```python
from build123d import *

# Parameters (mm, degrees)
EXTRUDE_1_DEPTH                    = 20
SKETCH_5_R                         = 0.7
EXTRUDE_3_DEPTH                    = 4
CUT_EXTRUDE_1_DEPTH                = 8.5
SKETCH_7_R                         = 0.65
EXTRUDE_4_DEPTH                    = 6.7
CHAMFER_1_SIZE                     = 0.3
PATTERN_LINEAR_2_COUNT             = 4
PATTERN_LINEAR_2_PITCH             = 5
PATTERN_LINEAR_3_COUNT             = 4
PATTERN_LINEAR_3_PITCH             = 5
CHAMFER_1_OF_PATTERN_LINEAR_3_SIZE = 0.3
EXTRUDE_5_DEPTH                    = 0.5
EXTRUDE_6_DEPTH                    = 0.5
CUT_EXTRUDE_2_REACH                = 28.613
SKETCH_10_W                        = 0.5
SKETCH_10_H                        = 8.5


with BuildPart() as part:
    # Эскиз1 → Вытянуть1 (new body)
    with BuildSketch(Plane(origin=(0, 0, 0), x_dir=(0, -1, 0), z_dir=(1, 0, 0))):
        Polygon((-9, 0), (-9, -0.5), (-12, 0), (-12, 8), (0, 8), (0, 0), align=None)
    extrude(amount=EXTRUDE_1_DEPTH)

    # Эскиз5 → Вытянуть3 (add)
    with BuildSketch(Plane(origin=(0, 8, -8), x_dir=(1, 0, 0), z_dir=(0, 0, 1))):
        with Locations((2.5, -6.5)):
            Circle(SKETCH_5_R)
    extrude_3 = extrude(amount=-EXTRUDE_3_DEPTH)

    # Эскиз6 → Вырез-Вытянуть1 (cut)
    with BuildSketch(Plane(origin=(0, 12, 0), x_dir=(1, 0, 0), z_dir=(0, 1, 0))):
        with BuildLine():
            Line((0, 6.5), (0, 1))
            Line((0, 1), (5, 1))
            Line((5, 1), (5, 6.5))
            ThreePointArc((5, 6.5), (2.5, 7.3), (0, 6.5))
        make_face()
    cut_extrude_1 = extrude(amount=-CUT_EXTRUDE_1_DEPTH, mode=Mode.SUBTRACT)

    # Эскиз7 → Вытянуть4 (add)
    with BuildSketch(Plane(origin=(0, 3.5, 0), x_dir=(1, 0, 0), z_dir=(0, 1, 0))):
        with Locations(Location((2.5, 4, 0), (0, 0, 90))):
            Circle(SKETCH_7_R)
    extrude_4 = extrude(amount=EXTRUDE_4_DEPTH)

    # Фаска1
    chamfer_1_edges = [part.edges().sort_by_distance(p)[0] for p in [
        (2.5, 10.2, -3.35),
    ]]
    chamfer(chamfer_1_edges, length=CHAMFER_1_SIZE)

    # Линейный массив2: Вытянуть3, Вырез-Вытянуть1 ×4
    with Locations(*[(i * PATTERN_LINEAR_2_PITCH, 0, 0) for i in range(1, PATTERN_LINEAR_2_COUNT)]):
        add(extrude_3)
        add(cut_extrude_1, mode=Mode.SUBTRACT)

    # Линейный массив3: Вытянуть4 ×4
    with Locations(*[(i * PATTERN_LINEAR_3_PITCH, 0, 0) for i in range(1, PATTERN_LINEAR_3_COUNT)]):
        add(extrude_4)

    # Фаска1 of Линейный массив3
    chamfer_1_of_pattern_linear_3_edges = [part.edges().sort_by_distance(p)[0] for p in [
        (7.5, 10.2, -3.35),
        (12.5, 10.2, -3.35),
        (17.5, 10.2, -3.35),
    ]]
    chamfer(chamfer_1_of_pattern_linear_3_edges, length=CHAMFER_1_OF_PATTERN_LINEAR_3_SIZE)

    # Эскиз8 → Вытянуть5 (add)
    with BuildSketch(Plane(origin=(20, 0, 0), x_dir=(0, 0, -1), z_dir=(1, 0, 0))):
        Polygon((0, 12), (8, 12), (8, 0), (0, 0), (0, 9), (-0.5, 9), align=None)
    extrude(amount=EXTRUDE_5_DEPTH)

    # Эскиз9 → Вытянуть6 (add)
    with BuildSketch(Plane.ZY):
        Polygon((-8, 12), (0, 12), (0.5, 9), (0, 9), (0, 0), (-8, 0), align=None)
    extrude(amount=EXTRUDE_6_DEPTH)

    # Эскиз10 → Вырез-Вытянуть2 (cut, up to next)
    with BuildSketch(Plane(origin=(0, 12, 0), x_dir=(1, 0, 0), z_dir=(0, 1, 0)), mode=Mode.PRIVATE) as cut_extrude_2_sk1:
        with Locations((20.25, 3.75)):
            Rectangle(SKETCH_10_W, SKETCH_10_H)
    cut_extrude_2_tool1 = extrude(cut_extrude_2_sk1.sketch, amount=-CUT_EXTRUDE_2_REACH, mode=Mode.PRIVATE) & part.part
    # Эскиз10 → Вырез-Вытянуть2 (cut, up to next)
    with BuildSketch(Plane(origin=(0, 12, 0), x_dir=(1, 0, 0), z_dir=(0, 1, 0)), mode=Mode.PRIVATE) as cut_extrude_2_sk2:
        with Locations((-0.25, 3.75)):
            Rectangle(SKETCH_10_W, SKETCH_10_H)
    cut_extrude_2_tool2 = extrude(cut_extrude_2_sk2.sketch, amount=-CUT_EXTRUDE_2_REACH, mode=Mode.PRIVATE) & part.part
    add(cut_extrude_2_tool1.solids().sort_by_distance((20.25, 12, -3.75))[0], mode=Mode.SUBTRACT)
    add(cut_extrude_2_tool2.solids().sort_by_distance((-0.25, 12, -3.75))[0], mode=Mode.SUBTRACT)


solid = part.part
```
Part model, mm, in its own coordinate system. A direction names the side the tool comes from. Give positions to 0.01 mm unless a question says otherwise; leave off trailing zeros. Order: outer loops, then holes, each group sorted by start corner. A loop starts at its lowest first (then second) coordinate and runs counter-clockwise, first axis right, second up. Notation, with made-up numbers: M 47,80.25 L 102,80.25 A25 cw 102,114.25 Z; hole C 56.25,48 d6. An arc over 180 degrees is marked long. Use a Markdown table: item, result. Add a question column.
(1) Drop flat-ended pins along their axis: P1, Ø1, axis at x = 15.5, y = 5.5, coming from the +Z side; P2, Ø0.8, axis at x = 12.5, z = -4, coming from the +Y side; P3, Ø1, axis at x = 13, z = -9.5, coming from the -Y side; P4, Ø5, axis at x = 5, z = -5, coming from the +Y side. Give the stop position or say it passes through.
(2) 3-axis set-ups, long thin cutter, end or side, ignore diameter. For faces 1 (the face through (10, 8, -1)), 2 (the face through (12.5, 7.8, -7.3)), 3 (the face through (13.147, 1.232, -9.972)): which of +Z, -Z, +X, -X, +Y, -Y reach the whole face in a straight line?
(3) Saw through at A-A, the plane y = 3.75. Give the cut face in (x, z), and give its area (3 significant figures).
(4) Saw through at D-D, the plane y = 1.5. Give the cut face in (x, z), and give its area (3 significant figures).
(5) Mould opens along X. For faces 4 (the face through (2.823, 0.879, -9.972)), 5 (the face through (10.1, 12, -0.5)), 6 (the face through (20, 3, -5)), 7 (the face through (7.3, 6.66, -4.62)) say: +X half, -X half, draft (parallel to the pull), parting line (faces both ways), or undercut.
(6) Probe line 1 along Z through (x, y) = (12.5, 7.25); line 2 along X through (y, z) = (4, -3.75); line 3 along Z through (x, y) = (19, 2.5). List the from-to ranges inside material, lowest first. Write a range as [from, to].
(7) Saw through at C-C, the plane z = -11. Give the cut face in (x, y), and give its area (3 significant figures).
(8) Saw through at B-B, the plane x = 2.5. Give the cut face in (y, z).
Answer key:
| question | item | result |
|---|---|---|
| 1 | P1 | z = 0 |
| 1 | P2 | y = 10.2 |
| 1 | P3 | y = 0.8 |
| 1 | P4 | y = 12 |
| 2 | face 1 | +X, -X, +Y |
| 2 | face 2 | +Y |
| 2 | face 3 | -Z |
| 3 | outline | M 0,-8 L 20,-8 L 20,-6.5 A4.31 cw 15,-6.5 A4.31 cw 10,-6.5 A4.31 cw 5,-6.5 A4.31 cw 0,-6.5 Z; M 0,-1 L 20,-1 L 20,0 L 0,0 Z; C 2.5,-4 d1.3; C 7.5,-4 d1.3; C 12.5,-4 d1.3; C 17.5,-4 d1.3 |
| 3 | area | 44.4 mm^2 |
| 4 | outline | M 0,-8 L 1.8,-8 L 1.8,-12 L 3.2,-12 L 3.2,-8 L 6.8,-8 L 6.8,-12 L 8.2,-12 L 8.2,-8 L 11.8,-8 L 11.8,-12 L 13.2,-12 L 13.2,-8 L 16.8,-8 L 16.8,-12 L 18.2,-12 L 18.2,-8 L 20,-8 L 20,0 L 0,0 Z |
| 4 | area | 182 mm^2 |
| 5 | face 4 | undercut |
| 5 | face 5 | draft |
| 5 | face 6 | +X half |
| 5 | face 7 | undercut |
| 6 | line 1 | [-8, -7.3], [-4.65, -3.35], [-1, 0] |
| 6 | line 2 | [1.9, 3.1], [6.9, 8.1], [11.9, 13.1], [16.9, 18.1] |
| 6 | line 3 | [-8, 0] |
| 7 | outline | C 2.5,1.5 d1.4; C 7.5,1.5 d1.4; C 12.5,1.5 d1.4; C 17.5,1.5 d1.4 |
| 7 | area | 6.16 mm^2 |
| 8 | outline | M 0,-8 L 0.8,-8 L 0.8,-12 L 2.2,-12 L 2.2,-8 L 12,-8 L 12,-7.3 L 3.5,-7.3 L 3.5,-4.65 L 9.9,-4.65 L 10.2,-4.35 L 10.2,-3.65 L 9.9,-3.35 L 3.5,-3.35 L 3.5,-1 L 12,-1 L 12,0 L 9,0.5 L 9,0 L 0,0 Z |
